The listing builds one solid part. Answer for the finished solid, in the listing's coordinates (mm). Give positions to 0.01 mm unless a question says otherwise; leave off trailing zeros. Loops run counter-clockwise (first coordinate to the right, second up) from the corner with the lowest first, then second, coordinate; pieces in that order, holes last. Notation, with made-up numbers: M 34,28.5 L 76,28.5 A20 ccw 76,61.5 Z; hole C 21.5,23.5 d2. An arc over 180 degrees is marked long. Use one line per item in the form item = value. Start each with the question number.
1. Straight lines are drawn through the part: line 1 (X direction, y = 25.4, z = -6.5); line 2 (Y direction, x = 0, z = -6.5); line 3 (Y direction, x = 0, z = -2.25). For each, find the intervals that lie inside material, in ascending order. Write a range as from..to.
2. Each of these flat-tipped pins is pushed along its axis until it touches: pin 1 Ø1.5 at (x, y) = (0, 25.4) entering from -Z; pin 2 Ø10 at (x, y) = (7, 59) entering from +Z; pin 3 Ø12 at (x, y) = (-3, 32.5) entering from -Z. Where does it stop, or does it pass through?
3. The part is cut by section B-B (y = 130). Write down the section's boundary in (x, z).
4. The part is cut by section A-A (x = 4.75). Write down the section's boundary in (y, z).
from build123d import *

# Parameters (mm, degrees)
BOSS_EXTRUDE1_DEPTH       = 12.7
F_0_80_TAPPED_HOLE1_D     = 1.19126
F_0_80_TAPPED_HOLE1_DEPTH = 10
F_0_80_TAPPED_HOLE1_TIP   = 0.357890611


with BuildPart() as part:
    # Sketch1 → Boss-Extrude1 (new body, symmetric)
    with BuildSketch(Plane(origin=(0, 0, 0), x_dir=(0, 0, -1), z_dir=(1, 0, 0))):
        Polygon((0, 0), (0, 50.8), (52.861, 142.357937739), (82.190393675, 142.357937739), align=None)
    extrude(amount=BOSS_EXTRUDE1_DEPTH, both=True)

    # #0-80 Tapped Hole1
    with Locations(Plane.XY):
        with Locations((0, 25.4)):
            Hole(F_0_80_TAPPED_HOLE1_D / 2, depth=F_0_80_TAPPED_HOLE1_DEPTH)
            with Locations((0, 0, -(F_0_80_TAPPED_HOLE1_DEPTH + F_0_80_TAPPED_HOLE1_TIP / 2))):  # 118° drill point
                Cone(0, F_0_80_TAPPED_HOLE1_D / 2, F_0_80_TAPPED_HOLE1_TIP, mode=Mode.SUBTRACT)


solid = part.part
Derived:
q1.line_1 = -12.7..-0.6, 0.6..12.7
q1.line_2 = 11.26..24.8, 26..62.06
q1.line_3 = 3.9..24.8, 26..54.7
q2.pin_1 = -15.1
q2.pin_2 = -1.85
q2.pin_3 = -22.23
q3.outline = M -12.7,-75.06 L 12.7,-75.06 L 12.7,-45.73 L -12.7,-45.73 Z
q4.outline = M 0,0 L 142.36,-82.19 L 142.36,-52.86 L 50.8,0 Z
